For this review, use the dimensioned drawing (mm, ordinates from the lowest corner) and the shaded views. A direction names the side the tool comes from. Coordinates: 2 decimals unless noted, no trailing zeros. Loops run counter-clockwise (first coordinate to the right, second up) from the corner with the lowest first, then second, coordinate; pieces in that order, holes last. Notation, with made-up numbers: (-12, -15) - (33, -15) arc R18 ccw to (33, 14) - close; hole circle Ø4 at (-37.75, 69). An arc over 180 degrees is marked (long way). One line per item, written item: value. Start each with the question number.
1. We need section A-A, the plane z = 48.5. Give the boundary of the cut face in (x, y), then the cut area to 3 significant figures.
2. For the marked faces 1 and 2, list the 3-axis set-ups (+Z, -Z, +X, -X, +Y, -Y) from which the entire face can be reached by the end or side of a thin tool; tool diameter is ignored.
3. We need section D-D, the plane y = 16. Give the boundary of the cut face in (x, z).
4. Insertion check: P1, Ø17, axis at y = 16, z = 48.5, coming from the +X side. The pin has a flat end and moves straight along its axis. Give the tip position at first contact, or say it passes through.
5. We need section C-C, the plane y = 5.5. Give the boundary of the cut face in (x, z).
6. To check wall thickness, follow line 1 (Y direction, x = 4.5, z = 144); line 2 (Y direction, x = 31.05, z = 48.5). State the ranges of each line that lie inside material, in increasing order.
7. We need section B-B, the plane x = 26.5. Give the boundary of the cut face in (y, z).
8. Mouldability with a two-part tool opening along Y and no side actions: class the marked faces 3, 4 and 5 as +Y half, -Y half, draft (parallel to the pull), parting line (faces both ways), or undercut.
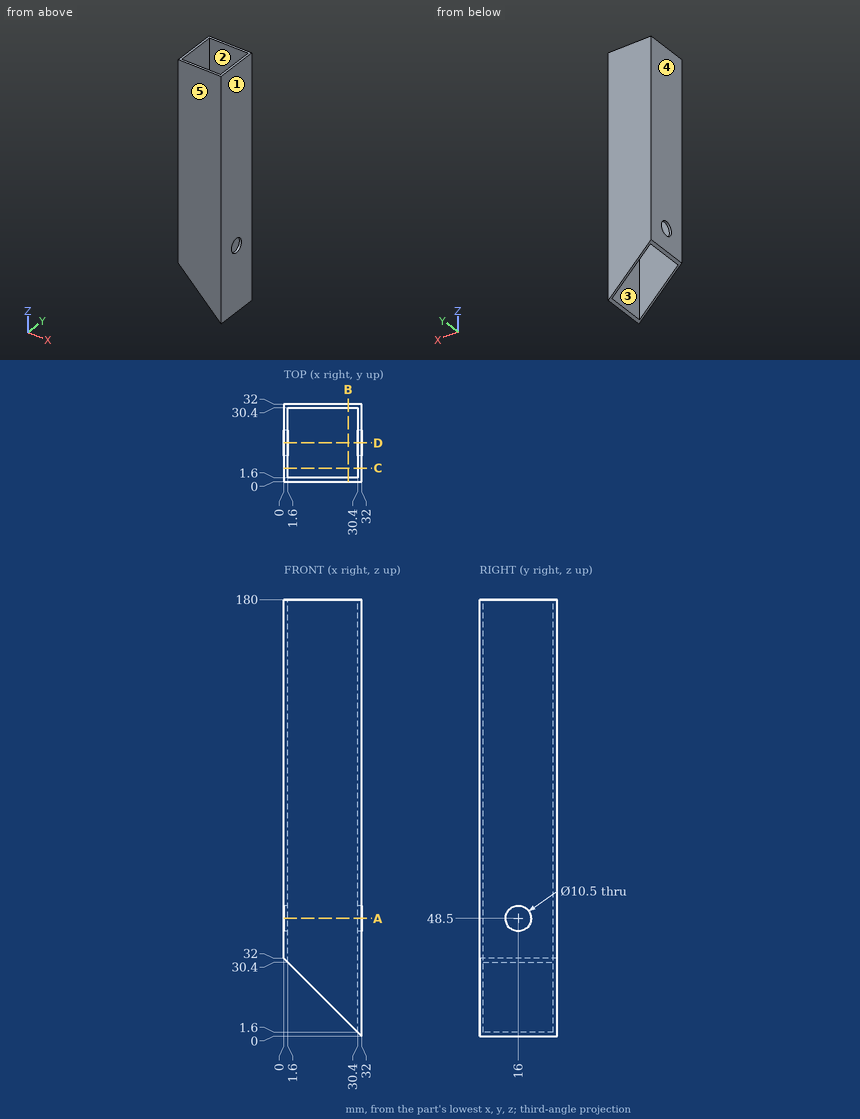
Findings below:
1. outline: (0, 0) - (32, 0) - (32, 10.75) - (30.4, 10.75) - (30.4, 1.6) - (1.6, 1.6) - (1.6, 10.75) - (0, 10.75) - close; (0, 21.25) - (1.6, 21.25) - (1.6, 30.4) - (30.4, 30.4) - (30.4, 21.25) - (32, 21.25) - (32, 32) - (0, 32) - close
1. area: 161 mm2
2. face 1: +Z, -Z, +X, +Y, -Y
2. face 2: +Z, -Z
3. outline: (0, 32) - (1.6, 30.4) - (1.6, 43.25) - (0, 43.25) - close; (0, 53.75) - (1.6, 53.75) - (1.6, 180) - (0, 180) - close; (30.4, 1.6) - (32, 0) - (32, 43.25) - (30.4, 43.25) - close; (30.4, 53.75) - (32, 53.75) - (32, 180) - (30.4, 180) - close
4. P1: x = 32
5. outline: (0, 32) - (1.6, 30.4) - (1.6, 180) - (0, 180) - close; (30.4, 1.6) - (32, 0) - (32, 180) - (30.4, 180) - close
6. line 1: 0 to 1.6, 30.4 to 32
6. line 2: 0 to 10.75, 21.25 to 32
7. outline: (0, 5.5) - (1.6, 5.5) - (1.6, 180) - (0, 180) - close; (30.4, 5.5) - (32, 5.5) - (32, 180) - (30.4, 180) - close
8. face 3: undercut
8. face 4: draft
8. face 5: -Y half
